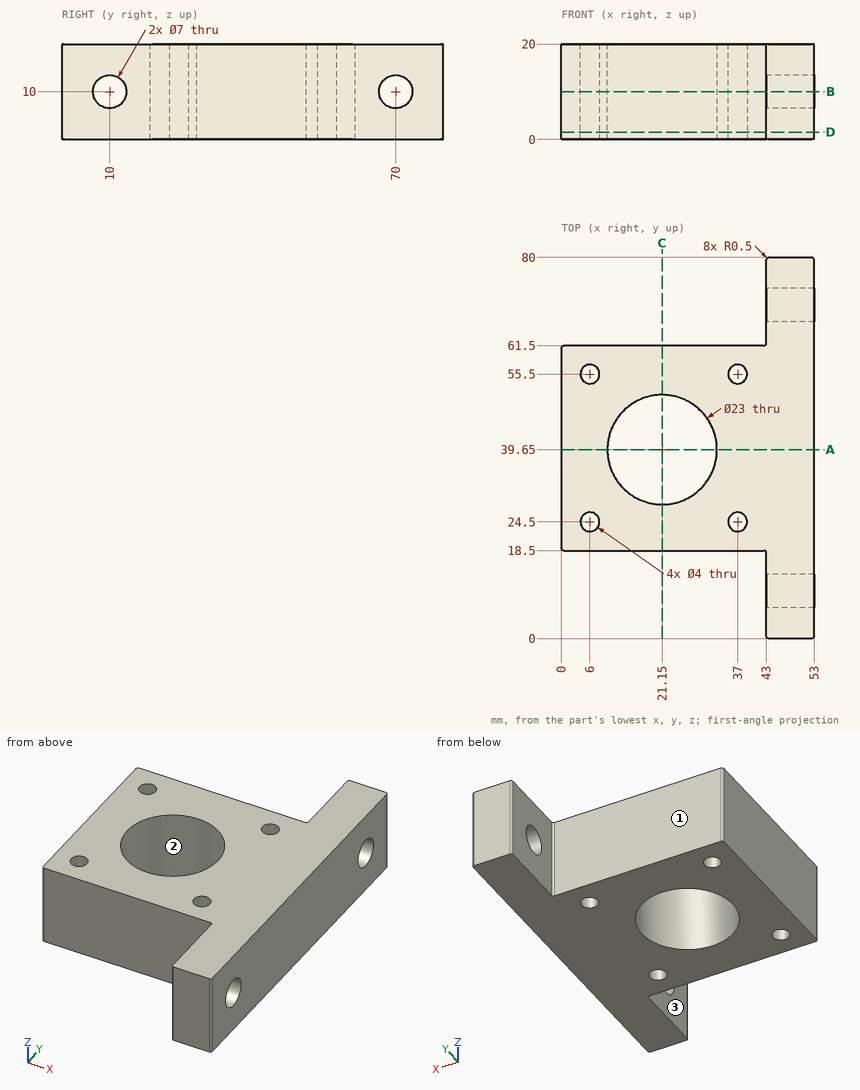
Here's the drawing with two shaded views (mm, measured from the low corner). I have some questions. A direction names the side the tool comes from. Coordinates: 2 decimals unless noted, no trailing zeros. Loops run counter-clockwise (first coordinate to the right, second up) from the corner with the lowest first, then second, coordinate; pieces in that order, holes last.
Item 1: Which directions (+Z, -Z, +X, -X, +Y, -Y) give clear straight access to the entire face, cutting with the end or side of a thin tool? Please do the marked faces 1, 2 and 3.
Answers below:
face 1: +Z, -Z, -X, +Y
face 2: +Z, -Z
face 3: +Z, -Z, -X, -Y
Item 2: I'm going to push flat-ended pins straight in: pin 1 (3 mm diameter, centred on x = 23.5, z = 13.5, fed in from -Y); pin 2 (5 mm diameter, centred on y = 75, z = 11.5, fed in from -X); pin 3 (3.5 mm diameter, centred on x = 6, y = 55.5, fed in from -Z); pin 4 (8 mm diameter, centred on x = 34, z = 11.5, fed in from +Y). Where does each tip first touch, or does it pass through?
Answers below:
pin 1: stops at y = 18.5
pin 2: stops at x = 43
pin 3: passes through
pin 4: stops at y = 61.5
Item 3: Suppose I cut it at A-A (y = 39.65). Please give me the cut outline in (x, z).
Answers below:
outline: (0, 0) - (9.65, 0) - (9.65, 20) - (0, 20) - close; (32.65, 0) - (53, 0) - (53, 20) - (32.65, 20) - close
Item 4: Suppose I cut it at C-C (x = 21.15). Please give me the cut outline in (y, z).
Answers below:
outline: (18.5, 0) - (28.15, 0) - (28.15, 20) - (18.5, 20) - close; (51.15, 0) - (61.5, 0) - (61.5, 20) - (51.15, 20) - close
Item 5: Please list where these lines run through material, in increasing order: L1, parallel to Y at x = 37, z = 10; L2, parallel to X at y = 24.5, z = 15.75; L3, parallel to Y at x = 47, z = 10.
Answers below:
L1: y = 18.5 to 22.5, 26.5 to 53.5, 57.5 to 61.5
L2: x = 0 to 4, 8 to 35, 39 to 53
L3: y = 0 to 6.5, 13.5 to 66.5, 73.5 to 80
Item 6: Suppose I cut it at D-D (z = 1.5). Please give me the cut outline in (x, y), then the cut area to 3 significant figures.
Answers below:
outline: (0, 19) arc R0.5 ccw to (0.5, 18.5) - (42.5, 18.5) arc R0.5 cw to (43, 18) - (43, 0.5) arc R0.5 ccw to (43.5, 0) - (52.5, 0) arc R0.5 ccw to (53, 0.5) - (53, 79.5) arc R0.5 ccw to (52.5, 80) - (43.5, 80) arc R0.5 ccw to (43, 79.5) - (43, 62) arc R0.5 cw to (42.5, 61.5) - (0.5, 61.5) arc R0.5 ccw to (0, 61) - close; hole circle Ø4 at (6, 24.5); hole circle Ø4 at (6, 55.5); hole circle Ø23 at (21.15, 39.65); hole circle Ø4 at (37, 24.5); hole circle Ø4 at (37, 55.5)
area: 2,180 mm2
Item 7: Suppose I cut it at B-B (z = 10). State how many separate pieces and enclosed holes the cut face has, then the cut area to 3 significant figures.
Answers below:
separate pieces: 3
enclosed holes: 5
area: 2,040 mm2
